Can you work these out from the model? Positions are in its coordinate system, mm. A direction names the side the tool comes from. Give positions to 0.01 mm unless a question says otherwise; leave off trailing zeros. Order: outer loops, then holes, each group sorted by start corner. A loop starts at its lowest first (then second) coordinate and runs counter-clockwise, first axis right, second up. Notation, with made-up numbers: (-25.75, -38.5) - (2.25, -38.5) arc R27 ccw to (2.25, -4.5) - close; hole circle Ø3 at (56, -3.75). An arc over 180 degrees is marked (long way). Answer as a JSON object with one key per item and string values.
Autodesk Inventor part; units mm, degrees
ref_plane "YZ Plane" through (0, 0, 0) normal (1, 0, 0) x (0, 1, 0)
ref_plane "XZ Plane" through (0, 0, 0) normal (0, 1, 0) x (-1, 0, 0)
ref_plane "XY Plane" through (0, 0, 0) normal (0, 0, 1) x (1, 0, 0)
sketch "Эскиз1" plane through (0, 0, 0) normal (0, 1, 0) x (-1, 0, 0)
  line L0 (0, -56) -> (0, -121)
  line L1 (0, -56) -> (-1, -56)
  line L2 (0, -56) -> (1, -56) construction
  line L3 (0, -121) -> (-1, -121)
  line L4 (0, -121) -> (1, -121) construction
  arc A0 (-1, -56) -> (-1, -121) centre (19.5, -88.5) ccw
  dimension "d5" = 65
  dimension "d6" = 1
  dimension "d7" = 180
  dimension "d8" = 1
  dimension "d9" = 180
extrude "Выдавливание1" add sketch "Эскиз1" along normal blind 4
sketch "Эскиз2" plane through (0, 4, 0) normal (0, 1, 0) x (1, 0, 0)
  line L0 (0, 121) -> (0, 56)
  line L1 (0, 56) -> (0, 121)
  line L2 (0, 121) -> (1, 121)
  line L3 (0, 56) -> (1, 56)
  arc A0 (1, 56) -> (1, 121) centre (-19.5, 88.5) ccw
  line L4 (5, 58.8985) -> (5, 118.1015)
  arc A1 (1, 56) -> (5, 58.8985) centre (-19.5, 88.5) ccw
  arc A2 (5, 118.1015) -> (1, 121) centre (-19.5, 88.5) ccw
  point P0 (0, 0)
extrude "Выдавливание2" add sketch "Эскиз2" along normal blind 16 contours L2 A0 L4 L3 L0
sketch "Эскиз3" plane through (0, 0, -121) normal (-1, 0, 0) x (0, 0, 1)
  line L0 (65, 0) -> (0, 0)
  line L1 (32.5, 0) -> (32.5, 20)
  line L2 (0, 20) -> (65, 20)
  line L3 (4.5, 10) -> (60.5, 10)
  circle A0 centre (4.5, 10) radius 2.25
  circle A1 centre (60.5, 10) radius 2.25
  point P0 (121, 0)
  dimension "d17" = 4.5
  dimension "d18" = 4.5
extrude "Выдавливание3" cut sketch "Эскиз3" against normal blind 5
sketch "Эскиз4" plane through (5, 4, -58.8985) normal (1, 0, 0) x (0, 0, -1)
  arc A0 (0, 4.4196) -> (0, 7.5804) centre (1.6015, 6) ccw
  circle A1 centre (1.6015, 6) radius 6
  line L0 (59.203, 0) -> (0, 0)
  arc A2 (59.203, 7.5804) -> (59.203, 4.4196) centre (57.6015, 6) ccw
  circle A3 centre (57.6015, 6) radius 6
  point P0 (-58.8985, -4)
extrude "Выдавливание4" cut sketch "Эскиз4" against normal blind 2
properties part number "05-01-Кронштейн низ защита (update)"
Q1. We'd pull the mould along Y, two halves only. Please class faces 1 (the face through (7, 0, -88)), 2 (the face through (3, 10, -114)), 3 (the face through (4.014, 9.822, -66.497)), 4 (the face through (5, 12, -88)): released by +Y, released by -Y, zero draft, split by the parting line, or undercut.
Recorded:
{"face 1": "released by -Y", "face 2": "undercut", "face 3": "undercut", "face 4": "zero draft"}
Q2. If we section it at A-A, the plane y = 10: Please give me the cut outline in (x, z), then the cut area to 3 significant figures.
Recorded:
{"outline": "(0, -121) - (1, -121) arc R38.43 ccw to (3, -119.65) - (3, -118.75) - (0, -118.75) - close; (0, -114.25) - (3, -114.25) - (3, -110.5) - (5, -110.5) - (5, -66.5) - (3, -66.5) - (3, -62.75) - (0, -62.75) - close; (0, -58.25) - (3, -58.25) - (3, -57.35) arc R38.43 ccw to (1, -56) - (0, -56) - close", "area": "253 mm^2"}
Q3. Which directions (+Z, -Z, +X, -X, +Y, -Y) give clear straight access to the entire face, cutting with the end or side of a thin tool? Please do faces 5 (the face through (0, 10, -88)), 6 (the face through (11, 4, -88)), 7 (the face through (4.014, 10.178, -110.503)).
Recorded:
{"face 5": "+Z, -Z, -X, +Y, -Y", "face 6": "+Z, -Z, +X, +Y", "face 7": "+X"}
Q4. If we section it at D-D, the plane z = -102: Please give me the cut outline in (x, y), then the cut area to 3 significant figures.
Recorded:
{"outline": "(0, 0) - (16.48, 0) - (16.48, 4) - (5, 4) - (5, 20) - (0, 20) - close", "area": "146 mm^2"}
Q5. If we section it at B-B, the plane y = 17.5: Please give me the cut outline in (x, z), then the cut area to 3 significant figures.
Recorded:
{"outline": "(0, -121) - (1, -121) arc R38.43 ccw to (5, -118.1) - (5, -58.9) arc R38.43 ccw to (1, -56) - (0, -56) - close", "area": "314 mm^2"}
Q6. I'm going to push flat-ended pins straight in: pin 1 Ø9.5 at (y, z) = (10, -116.5) entering from -X; pin 2 Ø5 at (y, z) = (10, -116.5) entering from +X; pin 3 Ø11 at (x, z) = (15.5, -96.5) entering from +Y. Where does each tip first touch, or does it pass through?
Recorded:
{"pin 1": "stops at x = 0", "pin 2": "stops at x = 3", "pin 3": "stops at y = 4"}
Q7. If we section it at C-C, the plane x = 2.25: Please give me the cut outline in (y, z), then the cut area to 3 significant figures.
Recorded:
{"outline": "(0, -120.18) - (20, -120.18) - (20, -56.82) - (0, -56.82) - close; hole circle Ø4.5 at (10, -116.5); hole circle Ø4.5 at (10, -60.5)", "area": "1,240 mm^2"}
Q8. I need wall thicknesses on L1, parallel to Y at x = 2.45, z = -116.5; L2, parallel to Z at x = 3.7, y = 10; L3, parallel to X at y = 8.75, z = -96. Which ranges of each line are inside material? Lowest first, please.
Recorded:
{"L1": "y = 0 to 7.75, 12.25 to 20", "L2": "z = -110.5 to -66.5", "L3": "x = 0 to 5"}
